Source: CAD feature listing. Evaluate the final solid. Frame: model axes, mm. A direction names the side the tool comes from. Coordinates: 2 decimals unless noted, no trailing zeros. Loops run counter-clockwise (first coordinate to the right, second up) from the corner with the lowest first, then second, coordinate; pieces in that order, holes last. Notation, with made-up numbers: (-24, 77) -> (-18, 77) arc R20 cw to (-18, 84) -> close; hole circle Ø6 at (-30.75, 86.25). An arc over 180 degrees is marked (long way). One line per question, with ' | ' between items. Start each with the question number.
```python
from build123d import *

# Parameters (mm, degrees)
F0_W     = 14
F0_H     = 9
F0_W_2   = 1
F0_W_3   = 16
F1_DEPTH = 1
F0_W_4   = 48
F0_H_2   = 11
F2_DEPTH = 71
F3_DEPTH = 71
F4_R     = 0.49999


# Not quite as in the source:
# - a fillet or chamfer is up to 0.001 mm smaller than in the source, because OpenCascade refuses the exact size


with BuildPart() as f1:
    # F0 (on Top) → F1 (new body)
    with BuildSketch(Plane.XY):
        with Locations((-11.0720558167, 5.5)):
            Rectangle(F0_W, F0_H)
        with Locations((-3.5720558167, 5.5)):
            Rectangle(F0_W_2, F0_H)
        with Locations((4.9279441833, 5.5)):
            Rectangle(F0_W_3, F0_H)
        with Locations((13.4279441833, 5.5)):
            Rectangle(F0_W_2, F0_H)
        with Locations((20.9279441833, 5.5)):
            Rectangle(F0_W, F0_H)
    extrude(amount=F1_DEPTH)

    # F0 (on Top) → F2 (join)
    with BuildSketch(Plane.XY):
        with Locations((4.9279441833, 5.5)):
            Rectangle(F0_W_4, F0_H_2)
        Polygon((-18.0720558167, 1), (-18.0720558167, 10), (-4.0720558167, 10), (-3.0720558167, 10), (12.9279441833, 10), (13.9279441833, 10), (27.9279441833, 10), (27.9279441833, 1), (13.9279441833, 1), (12.9279441833, 1), (-3.0720558167, 1), (-4.0720558167, 1), align=None, mode=Mode.SUBTRACT)
    extrude(amount=F2_DEPTH)

    # F0 (on Top) → F3 (join)
    with BuildSketch(Plane.XY):
        with Locations((-3.5720558167, 5.5)):
            Rectangle(F0_W_2, F0_H)
        with Locations((13.4279441833, 5.5)):
            Rectangle(F0_W_2, F0_H)
    extrude(amount=F3_DEPTH)

    # F4 (radius 0.5 in the source; OpenCascade refuses exactly that, so slightly less here)
    f4_edges = [f1.edges().sort_by_distance(p)[0] for p in [
        (-19.072056, 5.5, 71),
        (4.927944, 0, 71),
        (28.927944, 5.5, 71),
        (4.927944, 11, 71),
        (-18.072056, 5.5, 71),
        (-11.072056, 10, 71),
        (-4.072056, 5.5, 71),
        (-11.072056, 1, 71),
        (20.927944, 10, 71),
        (27.927944, 5.5, 71),
        (20.927944, 1, 71),
        (13.927944, 5.5, 71),
        (4.927944, 10, 71),
        (12.927944, 5.5, 71),
        (4.927944, 1, 71),
        (-3.072056, 5.5, 71),
        (28.927944, 11, 35.5),
        (-19.072056, 11, 35.5),
        (4.927944, 11, 0),
        (-19.072056, 0, 35.5),
        (-19.072056, 5.5, 0),
        (28.927944, 0, 35.5),
        (4.927944, 0, 0),
        (28.927944, 5.5, 0),
    ]]
    fillet(f4_edges, radius=F4_R)


solid = f1.part
```
(1) Draft query along X for faces 3 (the flat face through (28.928, 5, 35)), 4 (the flat face through (5, 11, 35)), 5 (the flat face through (27.928, 6, 35)). Return one class per face: pulls with the +X half, pulls with the -X half, needs draft (parallel to the pull), parting line crosses it, or undercut.
(2) Access query for faces 1 (the flat face through (21, 1, 35)), 2 (the flat face through (5, 6, 0)). Directions: +Z, -Z, +X, -X, +Y, -Y. A direction counts if a zero-diameter tool reaches every point of the face in a straight line with its end or side. Return the directions, or none.
(3) Cut plane A-A, the plane z = 12. Return the cut outline in (x, y), and give its area (3 significant figures).
(4) Ray query, L1, parallel to X at y = 8.5, z = 10.5; L2, parallel to Y at x = -10, z = 24.5; L3, parallel to Z at x = -15.5, y = 1.25. Return the intervals inside material, ascending.
(5) Contact query for a flat-ended pin moving along its axis: pin 1 Ø4.5 at (x, y) = (18, 3.5) entering from +Z. Output: stop coordinate, or through.
Here are the results:
1) face 3: pulls with the +X half | face 4: needs draft | face 5: undercut
2) face 1: +Z | face 2: -Z, +X, -X, +Y, -Y
3) outline: (-19.07, 0.5) arc R0.5 ccw to (-18.57, 0) -> (28.43, 0) arc R0.5 ccw to (28.93, 0.5) -> (28.93, 10.5) arc R0.5 ccw to (28.43, 11) -> (-18.57, 11) arc R0.5 ccw to (-19.07, 10.5) -> close; hole (-18.07, 1) -> (-4.07, 1) -> (-4.07, 10) -> (-18.07, 10) -> close; hole (-3.07, 1) -> (12.93, 1) -> (12.93, 10) -> (-3.07, 10) -> close; hole (13.93, 1) -> (27.93, 1) -> (27.93, 10) -> (13.93, 10) -> close | area: 132 mm2
4) L1: x = -19.07 to -18.07, -4.07 to -3.07, 12.93 to 13.93, 27.93 to 28.93 | L2: y = 0 to 1, 10 to 11 | L3: z = 0 to 1
5) pin 1: stops at z = 1
